from build123d import *

# Parameters (mm, degrees)
F0_R     = 11.05
F1_DEPTH = 8
F2_COUNT = 2
F3_F1_R  = 1
F3_F2_R  = 1


with BuildPart() as f1:
    # F0 (on Top) → F1 (new body)
    with BuildSketch(Plane.XY):
        with BuildLine():
            ThreePointArc((-10.0903869269, 14.2980450295), (-8.0519633873, -15.5375636961), (17.5, 0))
            ThreePointArc((17.5, 0), (14.3285222663, 10.0470617428), (5.9636057526, 16.4525197592))
            ThreePointArc((5.9636057526, 16.4525197592), (-2.3276642918, 17.3445086106), (-10.0903869269, 14.2980450295))
        make_face()
        Circle(F0_R, mode=Mode.SUBTRACT)
        with BuildLine():
            ThreePointArc((-10.0903869269, 14.2980450295), (-2.3276642918, 17.3445086106), (5.9636057526, 16.4525197592))
            Line((5.9636057526, 16.4525197592), (11.7946313694, 26.4485646039))
            Line((11.7946313694, 26.4485646039), (16.7984124273, 35.0264757872))
            Line((16.7984124273, 35.0264757872), (6.7908498459, 49.0847229958))
            Line((6.7908498459, 49.0847229958), (-7.5056743808, 49.0847229958))
            Line((-7.5056743808, 49.0847229958), (-15.6662040079, 35.0410211056))
            Line((-15.6662040079, 35.0410211056), (-10.0903869269, 14.2980450295))
        make_face()
        Polygon((-4.9219110448, 42.525), (4.9219110448, 42.525), (9.8438220897, 34), (4.9219110448, 25.475), (-4.9219110448, 25.475), (-9.8438220897, 34), align=None, mode=Mode.SUBTRACT)
    extrude(amount=F1_DEPTH)

    # F2: F1 ×2 about axis
    f2_axis = Axis((0, 0, 0), (0, 0, 1))


with BuildPart() as f1_1:
    add(f1.part)
    for i in range(1, F2_COUNT):
        add(f1.part.rotate(f2_axis, i * 360 / F2_COUNT))

    # F3: fillet of radius 1 on 31 edges, made by hand

    # F3_f1
    f3_f1_edges = [f1_1.edges().sort_by_distance(p)[0] for p in [
        (10.0903869269, -14.2980450295, 4),
        (5.9636057526, 16.4525197592, 4),
        (-10.0903869269, 14.2980450295, 4),
        (-5.9636057526, -16.4525197592, 4),
    ]]
    fillet(f3_f1_edges, radius=F3_F1_R)

    # F3_f2
    f3_f2_edges = [f1_1.edges().sort_by_distance(p)[0] for p in [
        (7.5056743808, -49.0847229958, 4),
        (15.6662040079, -35.0410211056, 4),
        (11.5859391943, -42.0628720507, 0),
        (11.5859391943, -42.0628720507, 8),
        (12.9670524021, -24.9997237726, 0),
        (12.9670524021, -24.9997237726, 8),
        (16.7984124273, 35.0264757872, 4),
        (11.6731868984, 26.2403740629, 0),
        (11.6731868984, 26.2403740629, 8),
        (6.7908498459, 49.0847229958, 4),
        (11.7946311366, 42.0555993915, 0),
        (11.7946311366, 42.0555993915, 8),
        (-7.5056743808, 49.0847229958, 4),
        (-0.3574122675, 49.0847229958, 0),
        (-0.3574122675, 49.0847229958, 8),
        (-15.6662040079, 35.0410211056, 4),
        (-11.5859391943, 42.0628720507, 0),
        (-11.5859391943, 42.0628720507, 8),
        (-12.9670524021, 24.9997237726, 0),
        (-12.9670524021, 24.9997237726, 8),
        (-16.7984124273, -35.0264757872, 4),
        (-11.6731868984, -26.2403740629, 0),
        (-11.6731868984, -26.2403740629, 8),
        (-6.7908498459, -49.0847229958, 4),
        (-11.7946311366, -42.0555993915, 0),
        (-11.7946311366, -42.0555993915, 8),
        (0.3574122675, -49.0847229958, 8),
        (-6.4610233416, -16.640341221, 8),
        (-6.4610233416, -16.640341221, 0),
        (-10.2868728829, 14.376857273, 8),
        (-10.2868728829, 14.376857273, 0),
        (6.4610233416, 16.640341221, 8),
        (6.4610233416, 16.640341221, 0),
        (10.2868728829, -14.376857273, 8),
        (10.2868728829, -14.376857273, 0),
    ]]
    fillet(f3_f2_edges, radius=F3_F2_R)


solid = f1_1.part
Part model, mm, in its own coordinate system. A direction names the side the tool comes from. Coordinates: 2 decimals unless noted, no trailing zeros. Loops run counter-clockwise (first coordinate to the right, second up) from the corner with the lowest first, then second, coordinate; pieces in that order, holes last. Notation, with made-up numbers: M 66,53 L 122,53 A27 ccw 122,86 Z; hole C -7.5,64.25 d8. An arc over 180 degrees is marked long. Use a Markdown table: item, result. Add a question column.
Q1. Cut at B-B (z = 5.5). Give the number of separate pieces and of enclosed holes in the cut face, and give its area (3 significant figures).
Q2. Probe L1, parallel to Y at x = 0, z = 2.5 (3 decimals); L2, parallel to Y at x = 1.5, z = 4 (3 decimals); L3, parallel to Y at x = -7.5, z = 1.5. List the from-to ranges inside material, lowest first.
Q3. Mould opens along Z. For faces 1 (the flat face through (-7.42, 38.2, 3.94)), 2 (the cylindrical face through (12.59, -24.74, 7.71)), 3 (the flat face through (3, -11, 0)) say: +Z half, -Z half, draft (parallel to the pull), parting line (faces both ways), or undercut.
Q4. Which spindle directions (+Z, -Z, +X, -X, +Y, -Y) get a long thin tool onto all of the face, cutting with end or side? Do faces 4 (the flat face through (-7.35, -38.32, 3.94)), 5 (the flat face through (-12.95, 24.94, 3.96)), 6 (the cylindrical face through (-12.59, 24.74, 0.29)). Say none if no direction does.
Q5. Cut at A-A (x = 0). Write the cut outline in (y, z) (3 decimals).
Q6. Pin check, flat tips, straight feed: P1, Ø3, axis at x = 12, z = 5, coming from the -Y side; P2, Ø4, axis at y = -15.5, z = 4, coming from the -X side; P3, Ø3, axis at y = 36.5, z = 1, coming from the +X side. Stop position of each tip, or through.
Worked out:
| question | item | result |
|---|---|---|
| 1 | separate pieces | 1 |
| 1 | enclosed holes | 3 |
| 1 | area | 1,640 mm2 |
| 2 | L1 | y = -49.085 to -42.525, -25.475 to -11.05, 11.05 to 25.475, 42.525 to 49.085 |
| 2 | L2 | y = -49.085 to -42.525, -25.475 to -10.948, 10.948 to 25.475, 42.525 to 49.085 |
| 2 | L3 | y = -48.09 to -38.06, -29.94 to -19.09, -15.81 to -8.11, 8.11 to 29.94, 38.06 to 48.91 |
| 3 | face 1 | draft |
| 3 | face 2 | +Z half |
| 3 | face 3 | -Z half |
| 4 | face 4 | +Z, -Z |
| 4 | face 5 | +Z, -Z, -X |
| 4 | face 6 | -Z, -X |
| 5 | outline | M -49.085,0 L -42.525,0 L -42.525,8 L -48.085,8 A1 ccw -49.085,7 Z; M -25.475,0 L -11.05,0 L -11.05,8 L -25.475,8 Z; M 11.05,0 L 25.475,0 L 25.475,8 L 11.05,8 Z; M 42.525,0 L 48.085,0 A1 ccw 49.085,1 L 49.085,7 A1 ccw 48.085,8 L 42.525,8 Z |
| 6 | P1 | stops at y = -43.93 |
| 6 | P2 | stops at x = -11.14 |
| 6 | P3 | stops at x = 16.61 |
